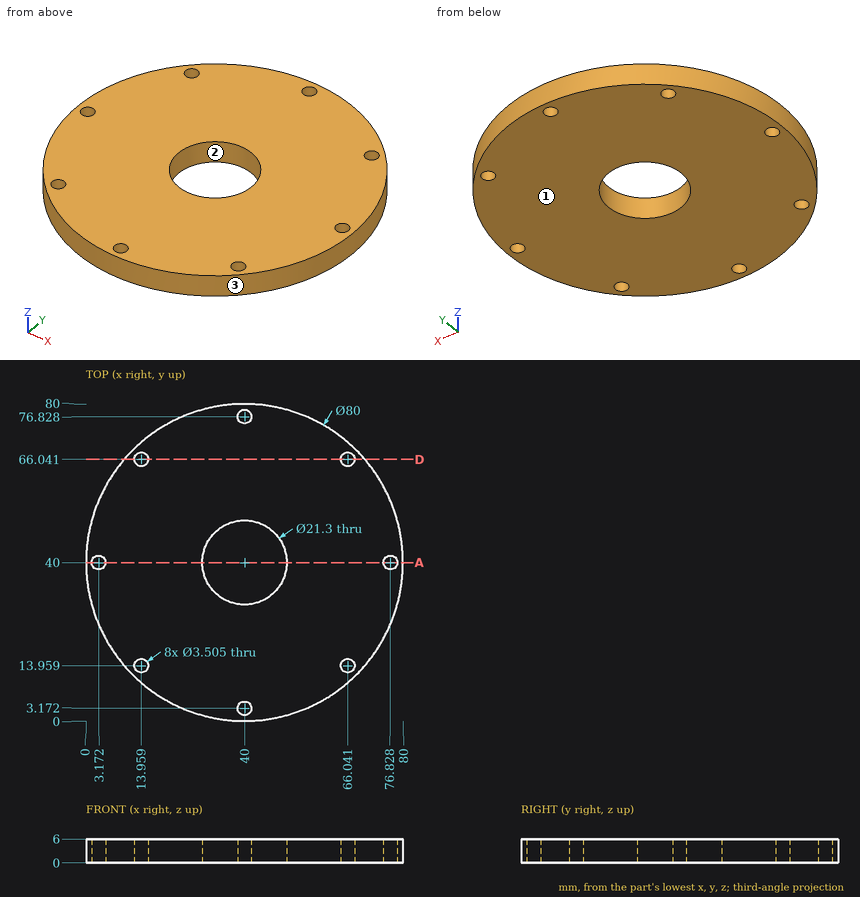
The drawing under review shows one solid part. Ordinate dimensions are in mm from its lowest x, y, z. Coordinates: 2 decimals unless noted, no trailing zeros. Order: outer loops, then holes, each group sorted by start corner. A loop starts at its lowest first (then second) coordinate and runs counter-clockwise, first axis right, second up. Notation, with made-up numbers: (14.25, 88.5) -> (42.25, 88.5) arc R32 ccw to (42.25, 122.5) -> close; hole circle Ø2 at (15.5, 10). An arc over 180 degrees is marked (long way). Answer in a Markdown table with one row per item. Add a question column.
Item 1: Mouldability with a two-part tool opening along X and no side actions: class the marked faces 1, 2 and 3 as +X half, -X half, draft (parallel to the pull), parting line (faces both ways), or undercut.
Item 2: We need section A-A on y = 40. Give the number of separate pieces and of enclosed holes in the cut face, plus the area to 3 significant figures.
Item 3: We need section D-D on y = 66. Write out the cut boundary in (x, z).
Item 4: Clearance check with a flat-ended pin moving along its axis: pin 1 (2 mm diameter, centred on x = 8.5, z = 3.5, fed in from -Y). State where the tip first meets the part, or that it passes through.
Item 5: To check wall thickness, follow probe 1 along X at (y, z) = (15.5, 4.05) (1 decimal); probe 2 along Y at (x, z) = (39.5, 3.25); probe 3 along Y at (x, z) = (48, 1.75). State the ranges of each line that lie inside material, in increasing order.
Final values:
| question | item | result |
|---|---|---|
| 1 | face 1 | draft |
| 1 | face 2 | undercut |
| 1 | face 3 | parting line |
| 2 | separate pieces | 4 |
| 2 | enclosed holes | 0 |
| 2 | area | 310 mm2 |
| 3 | outline | (9.6, 0) -> (12.21, 0) -> (12.21, 6) -> (9.6, 6) -> close; (15.71, 0) -> (64.29, 0) -> (64.29, 6) -> (15.71, 6) -> close; (67.79, 0) -> (70.4, 0) -> (70.4, 6) -> (67.79, 6) -> close |
| 4 | pin 1 | stops at y = 14.12 |
| 5 | probe 1 | x = 8.4 to 13.1, 14.8 to 65.2, 66.9 to 71.6 |
| 5 | probe 2 | y = 0 to 1.49, 4.85 to 29.36, 50.64 to 75.15, 78.51 to 80 |
| 5 | probe 3 | y = 0.81 to 32.97, 47.03 to 79.19 |
